from build123d import *

# Parameters (mm, degrees)
SKETCH1_W           = 47
SKETCH1_H           = 22.5
BOSS_EXTRUDE1_DEPTH = 2
BOSS_EXTRUDE2_DEPTH = 22.5


with BuildPart() as part:
    # Sketch1 → Boss-Extrude1 (new body)
    with BuildSketch(Plane(origin=(0, 0, 0), x_dir=(1, 0, 0), z_dir=(0, 1, 0))):
        Rectangle(SKETCH1_W, SKETCH1_H)
    extrude(amount=-BOSS_EXTRUDE1_DEPTH)

    # Sketch2 → Boss-Extrude2 (add)
    with BuildSketch(Plane.XY.offset(11.25)):
        Polygon((-23.5, 0), (23.5, 0), (23.5, 5), (15.5, 5), (15.5, 1.501741003), (-15.5, 1.501741003), (-15.5, 5), (-23.5, 5), align=None)
    extrude(amount=-BOSS_EXTRUDE2_DEPTH)


solid = part.part
Geometry check sheet. Reference: the model listing, model coordinates, mm. A direction names the side the tool comes from. Give positions to 0.01 mm unless a question says otherwise; leave off trailing zeros. Write each loop counter-clockwise with the first axis right and the second up, starting at its lowest first coordinate (ties: lowest second). Pieces come first, ordered by that corner, then holes. Notation, with made-up numbers: (47.5, 27) - (77.5, 27) arc R8 ccw to (77.5, 39) - close; hole circle Ø11 at (67.5, 59.5). An arc over 180 degrees is marked (long way). Put each result on its own line as item: value.
1. Sectioned sample at B-B, the plane z = -1. Enter the section's corners in (x, y), plus the area to 3 significant figures.
Ans:
outline: (-23.5, -2) - (23.5, -2) - (23.5, 5) - (15.5, 5) - (15.5, 1.5) - (-15.5, 1.5) - (-15.5, 5) - (-23.5, 5) - close
area: 221 mm²
2. Thickness scan on line 1 (X direction, y = 1.75, z = 1.75); line 2 (Y direction, x = 1.5, z = -8.5). Record the ranges inside material, lowest first.
Ans:
line 1: x = -23.5 to -15.5, 15.5 to 23.5
line 2: y = -2 to 1.5
3. Draft check along X on faces 3 (the flat face through (-15.5, 3, 0)), 4 (the flat face through (20, 5, 0)), 5 (the flat face through (-23.5, 2, 0)), 6 (the flat face through (23.5, 1, 0)). Enter one of: +X half, -X half, draft (parallel to the pull), parting line (faces both ways), or undercut.
Ans:
face 3: undercut
face 4: draft
face 5: -X half
face 6: +X half
4. Go/stop test with a flat-tipped pin: pin 1 (2 mm diameter, centred on x = -6, z = -1.5, fed in from +Y). Record where the tip stops, or that it passes through.
Ans:
pin 1: stops at y = 1.5
5. Sectioned sample at C-C, the plane x = -9. Enter the section's corners in (y, z), plus the area to 3 significant figures.
Ans:
outline: (-2, -11.25) - (1.5, -11.25) - (1.5, 11.25) - (-2, 11.25) - close
area: 78.8 mm²
6. Sectioned sample at A-A, the plane y = 2. Enter the section's corners in (x, z), plus the area to 3 significant figures.
Ans:
outline: (-23.5, -11.25) - (-15.5, -11.25) - (-15.5, 11.25) - (-23.5, 11.25) - close; (15.5, -11.25) - (23.5, -11.25) - (23.5, 11.25) - (15.5, 11.25) - close
area: 360 mm²
7. Set-up check for faces 1 (the flat face through (0, 1, -11.25)), 2 (the flat face through (0, 1.502, 0)): record each of +Z, -Z, +X, -X, +Y, -Y from which the full face is reachable in a straight line by a thin tool's end or side.
Ans:
face 1: -Z, +X, -X, +Y, -Y
face 2: +Z, -Z, +Y
